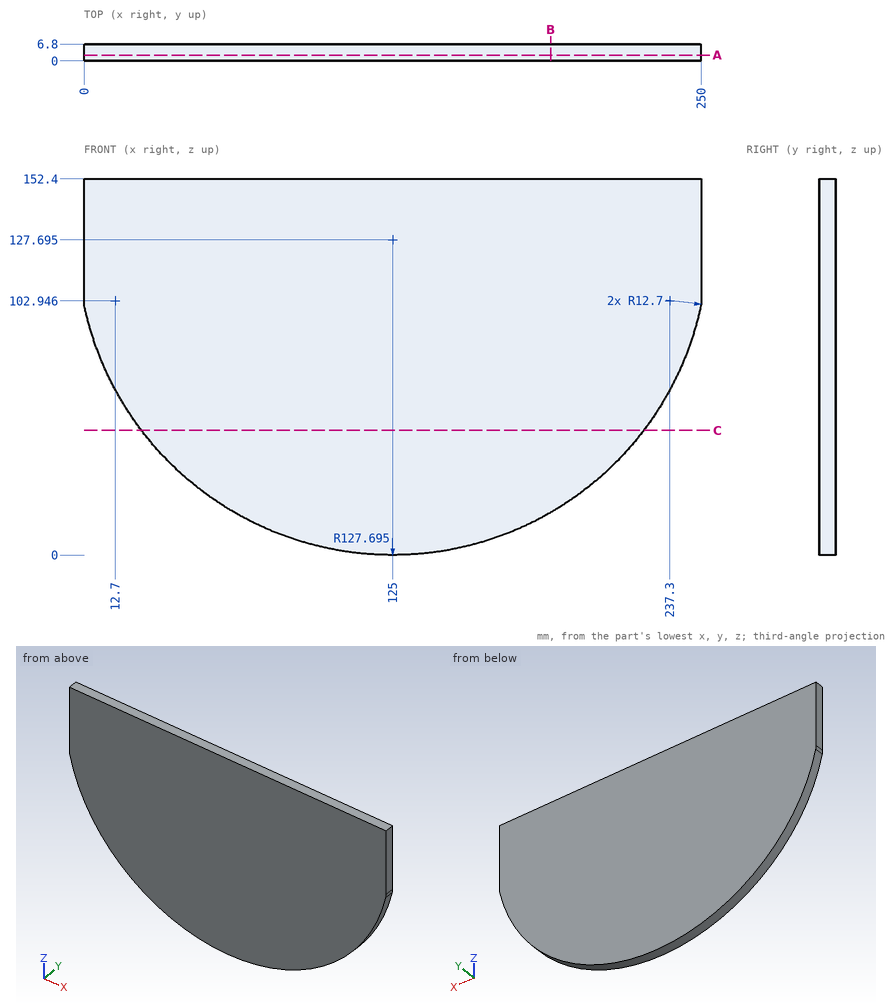
Verification items for this drawing (mm, ordinates from the low corner). Coordinates: 2 decimals unless noted, no trailing zeros. Order: outer loops, then holes, each group sorted by start corner. A loop starts at its lowest first (then second) coordinate and runs counter-clockwise, first axis right, second up.
Q1. Sectioned sample at A-A on y = 2.25. Record the cut outline in (x, z) (1 decimal).
Reply:
outline: (0, 102.9) arc R12.7 ccw to (0.3, 100.2) arc R127.7 ccw to (249.7, 100.2) arc R12.7 ccw to (250, 102.9) - (250, 152.4) - (0, 152.4) - close
Q2. Sectioned sample at C-C on z = 50.5. Record the cut outline in (x, y), and give its area (3 significant figures).
Reply:
outline: (23.28, 0) - (226.72, 0) - (226.72, 6.8) - (23.28, 6.8) - close
area: 1,380 mm2
Q3. Depth check by flat-ended pin: pin 1 Ø1 at (y, z) = (3.5, 37.5) entering from -X; pin 2 Ø2 at (y, z) = (5.5, 41.5) entering from +X. Enter the tip coordinate at first touch or a pass-through.
Reply:
pin 1: stops at x = 34.11
pin 2: stops at x = 220.12
Q4. Thickness scan on probe 1 along X at (y, z) = (5.5, 86.5); probe 2 along Z at (x, y) = (74.5, 5); probe 3 along X at (y, z) = (5, 52). Record the ranges inside material, lowest first.
Reply:
probe 1: x = 4.13 to 245.87
probe 2: z = 10.41 to 152.4
probe 3: x = 22.16 to 227.84
Q5. Sectioned sample at B-B on x = 189. Record the cut outline in (y, z).
Reply:
outline: (0, 17.2) - (6.8, 17.2) - (6.8, 152.4) - (0, 152.4) - close
